Autodesk Inventor part; units mm, degrees
ref_plane "Slot Start Plane" through (0, 0, -1.7245) normal (0, 0, 1) x (1, 0, 0)
ref_plane "YZ Plane" through (0, 0, 0) normal (1, 0, 0) x (0, 1, 0)
ref_plane "XZ Plane" through (0, 0, 0) normal (0, 1, 0) x (-1, 0, 0)
ref_plane "Slot Start Plane" through (0, 0, -1.7245) normal (0, 0, 1) x (1, 0, 0)
sketch "Key Profile" plane through (0, 0, 0) normal (1, 0, 0) x (0, 1, 0)
  line L0 (-2, 2.8563) -> (0.684, 1.8794)
  arc A0 (1.6188, -1.1745) -> (0.684, 1.8794) centre (0, 0) ccw
  line L1 (-2, 1.3132) -> (0.1881, 0.5168)
  arc A1 (0, -0.55) -> (0.1881, 0.5168) centre (0, 0) ccw
  line L2 (-2, 2.8563) -> (-2, -0.55)
  line L3 (0, 0) -> (-2, 0) construction
  line L4 (0, -0.55) -> (-2, -0.55)
  line L5 (1.6188, -1.1745) -> (-0.097, -0.55)
  line L6 (6, -5.55) -> (6, 87.7952)
  line L7 (-2, 87.9773) -> (-2, 2.8563)
  arc A2 (6, 87.7952) -> (-2, 87.9773) centre (0, 0) ccw
  line L8 (-2, -0.55) -> (-2, -7.55)
  arc A3 (4, -7.55) -> (6, -5.55) centre (4, -5.55) ccw
  line L9 (-2, -7.55) -> (4, -7.55)
  arc A4 (6, 55.1747) -> (-2, 55.464) centre (0, 0) ccw
  arc A5 (-2, 2.8563) -> (-2, 83.2148) centre (-539.3737, 43.0355) ccw
  point P0 (-0.5, 43.0355)
  point P1 (-0.6441, 55.4963)
  dimension "my_hingeCutRad" = 0.55
  dimension "my_hingeDepth" = 2
  dimension "my_hingeRegCutRad" = 2
  dimension "keyLength" = 88
  dimension "my_KeyHeight" = 8
  dimension "d107" = 20
  dimension "d122" = 4
  dimension "slotOffset" = 1.1745
  dimension "my_backWidth" = 7
  dimension "d128" = 55.5
  dimension "d135" = 1.5
  dimension "d136" = 4.7625
extrude "Upper (u)" add sketch "Key Profile" along normal blind 13.4643 and the other way blind 6.6071 contours A5 A4 L6 A3 L9 L8 L4 L5 A0 L0 | L0 A0 L5 L4 A1 L1 L2
extrude "Lower (d)" add sketch "Key Profile" along normal blind 13.4643 and the other way blind 6.6071 contours A5 L7 A2 L6 A4
extrude "Protrusion Cutout" cut sketch "Key Profile" along normal mid plane 4.5 contours L0 A0 L5 L4 A1 L1 L2
fillet "Front Fillet" radius 1.5 1 edges at (3.4286, 6, 87.7952)
sketch "Slot Sketch" plane through (0, 0, -1.7245) normal (0, 0, 1) x (1, 0, 0)
  line L0 (2.15, -2) -> (2.15, 1)
  line L1 (3.1, 4) -> (-3.1, 4)
  line L2 (-2.15, 1) -> (-2.15, -2)
  line L3 (-2.15, -2) -> (2.15, -2)
  line L4 (0, -2) -> (0, 4) construction
  line L5 (-3.1, 4) -> (-3.1, 1)
  line L6 (-3.1, 1) -> (-2.15, 1)
  line L7 (2.15, 1) -> (3.1, 1)
  line L8 (3.1, 1) -> (3.1, 4)
  point P0 (0, 0)
  dimension "d109" = 2
  dimension "my_slotHeadOffset" = 1
  dimension "my_slotHeadHeight" = 3
  dimension "my_slotHeadWidth" = 6.2
  dimension "my_neckSlotWidth" = 4.3
extrude "Slot" cut sketch "Slot Sketch" against normal through all
fillet "Edge Softening" radius 0.7 10 edges at (13.4643, 5.4142, -6.9642) (13.4643, 1, -7.55) (13.4643, 6, 40.4164) (-6.6071, 5.4142, -6.9642) (-6.6071, 1, -7.55) (-6.6071, 6, 40.4164) (-6.6071, 5.5879, 87.4156) (-6.6071, 1.2899, 87.9905) (13.4643, 5.5879, 87.4156) (13.4643, 1.2899, 87.9905)
equation "\"my_headHeight\" = 3"
equation "\"my_headOffset\" = 1"
equation "\"whiteKeyWidth\" = 20.07143"
properties part number "CKey0_Top"
Geometry: final body of the model. Coordinates: model frame, mm. A direction names the side the tool comes from. Coordinates: 2 decimals unless noted, no trailing zeros. Loops run counter-clockwise (first coordinate to the right, second up) from the corner with the lowest first, then second, coordinate; pieces in that order, holes last. Notation, with made-up numbers: M 70,43 L 76,43 A8 cw 76,53 Z; hole C -17.75,-29 d5. An arc over 180 degrees is marked long. One line per item, written item: value. Start each with the question number.
1) Pin query (flat end, axial travel): P1, Ø1.8, axis at x = 1, y = 1.5, coming from the -Z side. Return the tip coordinate at first contact, or that it passes through.
2) Cut plane A-A (x = 9). Return loops of the section in (y, z).
3) Draft query along Y for faces 5 (the cylindrical face through (-0.031, 1.905, 0.61)), 6 (the flat face through (2.15, -1, -5)), 7 (the cylindrical face through (3.3, 5.43, -6.95)). Return one class per face: released by +Y, released by -Y, zero draft, split by the parting line, or undercut.
4) Cut plane D-D (z = 13). Return loops of the section in (x, y), then the cut area to 3 significant figures.
5) Material intervals for L1, parallel to Z at x = 11.75, y = -0.25; L2, parallel to Z at x = 10, y = 1.5; L3, parallel to Y at x = 2.5, z = 16, sorted ascending. Write a range as from..to.
6) Cut plane B-B (z = 45.5). Return loops of the section in (x, y), then the cut area to 3 significant figures.
7) Cut plane C-C (x = 0). Return loops of the section in (y, z).
8) Reachability of faces 1 (the flat face through (0, 4, -5)), 2 (the flat face through (-0.031, -0.677, 2.375)), 3 (the flat face through (-2.15, 0, -5)), 4 (the flat face through (-4.46, -0.92, 0.92)) from +Z, -Z, +X, -X, +Y, -Y: full face, straight path, thin tool, end or side. Return the list, or none.
Evaluation:
1. P1: z = -1.72
2. outline: M -2,-7.55 L 4,-7.55 A2 ccw 6,-5.55 L 6,86.38 A1.5 ccw 4.58,87.88 A88.02 ccw -2,87.98 L -2,83.21 A538.88 cw -2,2.86 L -2,1.31 L 0.19,0.52 A0.55 cw 0,-0.55 L -2,-0.55 Z
3. face 5: undercut
3. face 6: zero draft
3. face 7: released by +Y
4. outline: M -6.61,-1.34 L 13.46,-1.34 L 13.46,5.3 A0.7 ccw 12.76,6 L -5.91,6 A0.7 ccw -6.61,5.3 Z
4. area: 147 mm^2
5. L1: -7.55..-0.55, 0.68..88
5. L2: -7.55..87.99
5. L3: -1.18..6
6. outline: M -6.61,-0.51 L 13.46,-0.51 L 13.46,5.3 A0.7 ccw 12.76,6 L -5.91,6 A0.7 ccw -6.61,5.3 Z
6. area: 130 mm^2
7. outline: M -2,-1.72 L 4,-1.72 L 4,-7.55 A2 ccw 6,-5.55 L 6,86.38 A1.5 ccw 4.58,87.88 A88.02 ccw -2,87.98 L -2,83.21 A538.88 cw -2,2.86 L 0.68,1.88 A2 cw 1.62,-1.17 L -0.1,-0.55 L -2,-0.55 Z
8. face 1: -Z
8. face 2: -Y
8. face 3: -Z, -Y
8. face 4: +X, -X, -Y
